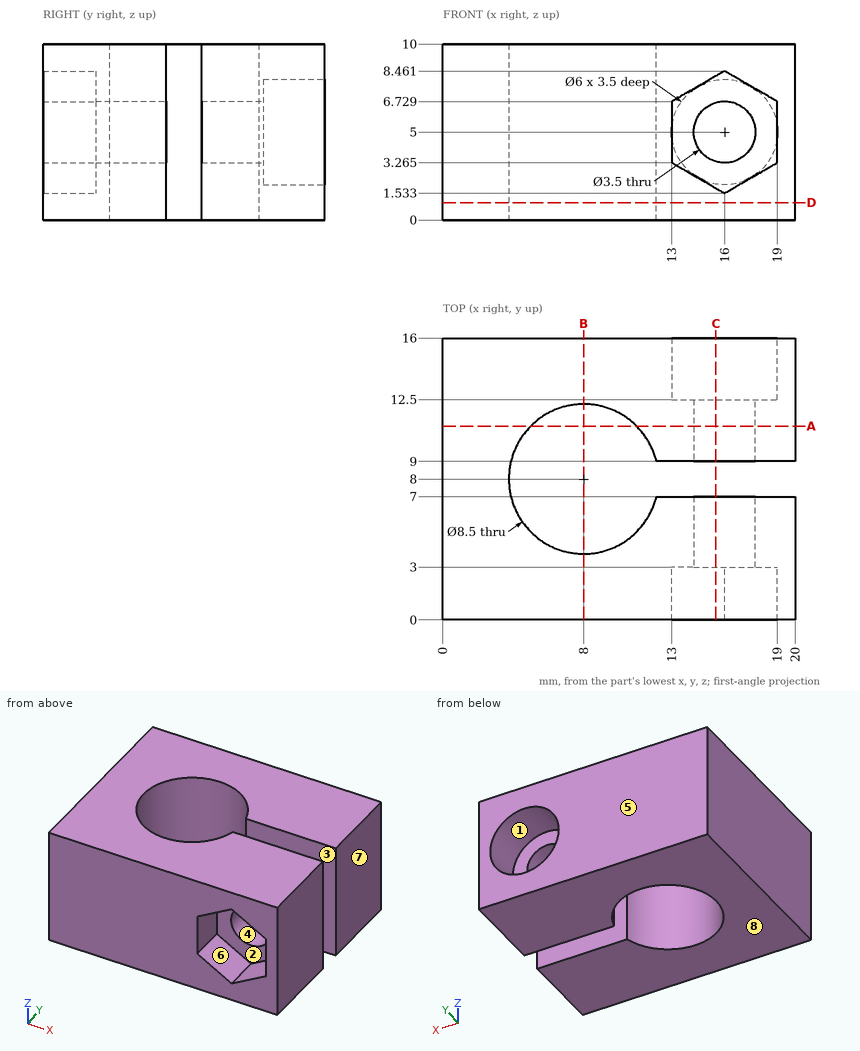
Study the drawing (mm; zero at the part's minimum x, y, z) and answer. A direction names the side the tool comes from. Coordinates: 2 decimals unless noted, no trailing zeros. Write each loop counter-clockwise with the first axis right and the second up, starting at its lowest first coordinate (ties: lowest second). Pieces come first, ordered by that corner, then holes. Notation, with made-up numbers: M 4.5,1.5 L 48.5,1.5 A20 cw 48.5,19.5 Z; hole C 75.25,-15 d1. An arc over 180 degrees is marked long. Use a Markdown table: item, result. Add a question column.
1. For a pull along X with two mould halves and no side action, classify the marked faces 6, 7 and 8 as +X half, -X half, draft (parallel to the pull), parting line (faces both ways), or undercut.
2. Section A-A (y = 11) is taken. Give the vertices of the cut face in (x, z).
3. Section B-B (x = 8) is taken. Give the vertices of the cut face in (y, z), plus the area to 3 significant figures.
4. Section C-C (x = 15.5) is taken. Give the vertices of the cut face in (y, z).
5. Straight lines are drawn through the part: line 1 along Y through (x, z) = (8, 8); line 2 along Z through (x, y) = (16, 5.75); line 3 along Z through (x, y) = (16, 14). For each, find the intervals that lie inside material, in ascending order. Write a range as [from, to].
6. Given P1, Ø5, axis at x = 14.5, z = 3.5, coming from the +Y side, flat-ended and moving along its own axis, determine where the tip first touches the part or whether it passes through.
7. Which of the six approach directions +Z, -Z, +X, -X, +Y, -Y give full straight-line access (tool end or side, diameter ignored) to the marked faces 1, 2, 3, 4 and 5?
8. Section D-D (z = 1) is taken. Give the vertices of the cut face in (x, y), plus the area to 3 significant figures.
Data:
| question | item | result |
|---|---|---|
| 1 | face 6 | undercut |
| 1 | face 7 | +X half |
| 1 | face 8 | draft |
| 2 | outline | M 0,0 L 4.99,0 L 4.99,10 L 0,10 Z; M 11.01,0 L 20,0 L 20,10 L 11.01,10 Z; hole C 16,5 d3.5 |
| 3 | outline | M 0,0 L 3.75,0 L 3.75,10 L 0,10 Z; M 12.25,0 L 16,0 L 16,10 L 12.25,10 Z |
| 3 | area | 75.0 mm2 |
| 4 | outline | M 0,0 L 7,0 L 7,3.32 L 3,3.32 L 3,1.82 L 0,1.82 Z; M 0,8.17 L 3,8.17 L 3,6.68 L 7,6.68 L 7,10 L 0,10 Z; M 9,0 L 16,0 L 16,2.04 L 12.5,2.04 L 12.5,3.32 L 9,3.32 Z; M 9,6.68 L 12.5,6.68 L 12.5,7.96 L 16,7.96 L 16,10 L 9,10 Z |
| 5 | line 1 | y = [0, 3.75], [12.25, 16] |
| 5 | line 2 | z = [0, 3.25], [6.75, 10] |
| 5 | line 3 | z = [0, 2], [8, 10] |
| 6 | P1 | stops at y = 16 |
| 7 | face 1 | +Y |
| 7 | face 2 | -Y |
| 7 | face 3 | +Z, -Z, +X |
| 7 | face 4 | +Y, -Y |
| 7 | face 5 | +Z, -Z, +X, -X, +Y |
| 8 | outline | M 0,0 L 20,0 L 20,7 L 12.13,7 A4.25 cw long 12.13,9 L 20,9 L 20,16 L 0,16 Z |
| 8 | area | 248 mm2 |
